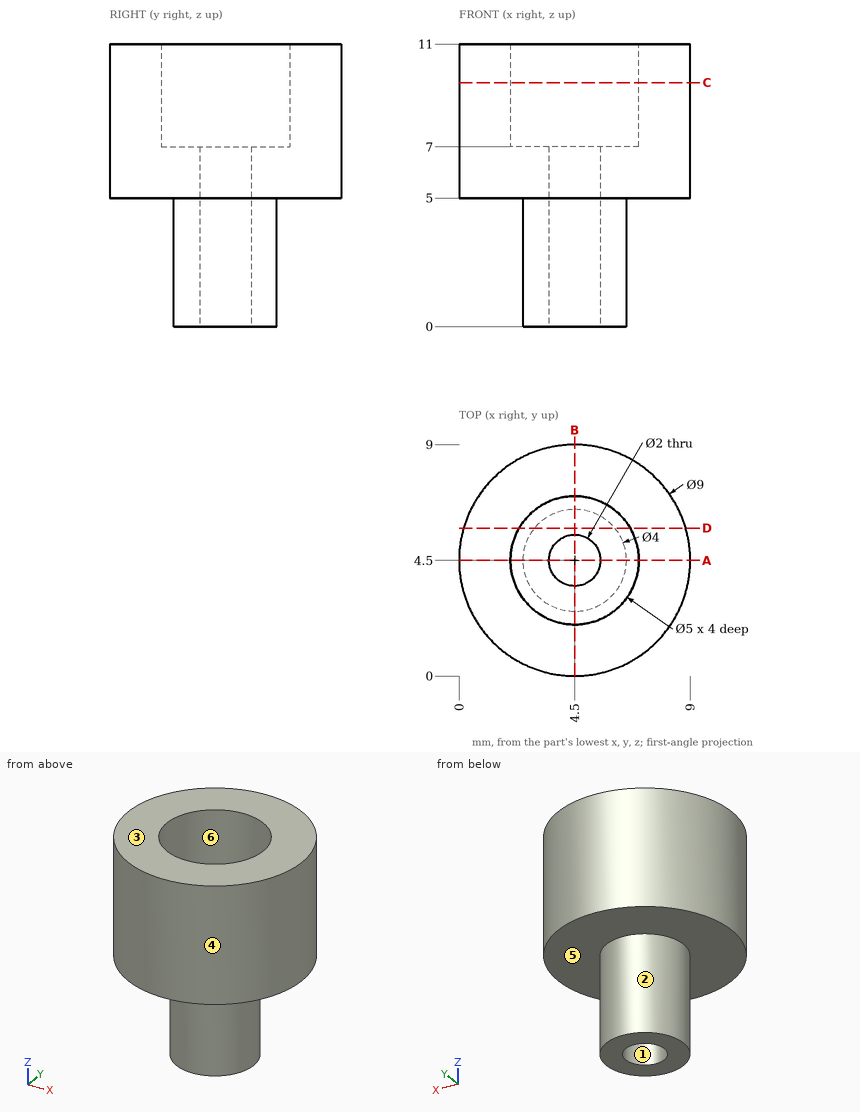
Here's the drawing with two shaded views (mm, measured from the low corner). I have some questions. A direction names the side the tool comes from. Round coordinates to 2 decimals unless told otherwise and drop trailing zeros. Loops run counter-clockwise (first coordinate to the right, second up) from the corner with the lowest first, then second, coordinate; pieces in that order, holes last. Notation, with made-up numbers: (-4, 56.25) - (8, 56.25) arc R11 cw to (8, 76.25) - close; hole circle Ø9 at (18, 5). An arc over 180 degrees is marked (long way). Use CSV: the item, a comma, the result in double quotes. Start each with the question number.
1) For pin 1 Ø5 at (x, z) = (8, 4) entering from +Y; pin 2 Ø4.5 at (x, y) = (4.5, 4.5) entering from +Z; pin 3 Ø5 at (y, z) = (7, 3) entering from -X, each with a flat end and sliding along its axis, tell me the tip position at first contact or that it passes through.
2) Please list where these lines run through material, in increasing order: probe 1 along X at (y, z) = (4.5, 3); probe 2 along Y at (x, z) = (4.5, 8.2). Write a range as [from, to].
3) If we section it at D-D on y = 5.75: Write out the boundary of the cut face in (x, z), plus the area to 3 significant figures.
4) For the marked faces 4, 5 and 6, which set-ups out of +Z, -Z, +X, -X, +Y, -Y let a thin tool reach every point of the face, with its end or its side?
5) We'd pull the mould along Y, two halves only. Please class the marked faces 1, 2 and 3: released by +Y, released by -Y, zero draft, split by the parting line, or undercut.
6) If we section it at A-A on y = 4.5: Write out the boundary of the cut face in (x, z).
7) If we section it at C-C on z = 9.5: Write out the boundary of the cut face in (x, y), plus the area to 3 significant figures.
Geometry results:
1,pin 1,"stops at y = 8.83"
1,pin 2,"stops at z = 7"
1,pin 3,"stops at x = 0.11"
2,probe 1,"x = [2.5, 3.5], [5.5, 6.5]"
2,probe 2,"y = [0, 2], [7, 9]"
3,outline,"(0.18, 5) - (2.94, 5) - (2.94, 0) - (6.06, 0) - (6.06, 5) - (8.82, 5) - (8.82, 11) - (6.67, 11) - (6.67, 7) - (2.33, 7) - (2.33, 11) - (0.18, 11) - close"
3,area,"50.2 mm2"
4,face 4,"+Z, -Z"
4,face 5,"-Z"
4,face 6,"+Z"
5,face 1,"undercut"
5,face 2,"split by the parting line"
5,face 3,"zero draft"
6,outline,"(0, 5) - (2.5, 5) - (2.5, 0) - (3.5, 0) - (3.5, 7) - (2, 7) - (2, 11) - (0, 11) - close; (5.5, 0) - (6.5, 0) - (6.5, 5) - (9, 5) - (9, 11) - (7, 11) - (7, 7) - (5.5, 7) - close"
7,outline,"circle Ø9 at (4.5, 4.5); hole circle Ø5 at (4.5, 4.5)"
7,area,"44.0 mm2"
